Autodesk Inventor part; units mm, degrees
ref_plane "YZ Plane" through (0, 0, 0) normal (1, 0, 0) x (0, 1, 0)
ref_plane "XZ Plane" through (0, 0, 0) normal (0, 1, 0) x (-1, 0, 0)
ref_plane "XY Plane" through (0, 0, 0) normal (0, 0, 1) x (1, 0, 0)
sketch "スケッチ1" plane through (0, 0, 0) normal (0, 0, 1) x (1, 0, 0)
  circle A0 centre (295.848871, -93.120076) radius 1.5
  circle A1 centre (295.848871, -93.120076) radius 3.025
  line L0 (302.911618, -92.777137) -> (291.344796, -101.566309)
  arc A2 (282.40584, -101.176779) -> (291.344796, -101.566309) centre (287.109706, -95.992799) ccw
  arc A3 (299.078829, -95.689522) -> (299.346701, -89.542385) centre (296.658778, -92.504659) ccw
  line L1 (214.413679, -12.475426) -> (302.911618, -92.777137)
  line L2 (186.870748, -14.489658) -> (289.472001, -107.588508)
  line L3 (89.513673, -53) -> (377.048162, -53)
  circle A4 centre (295.848871, -93.120076) radius 4.025
  circle A5 centre (295.848871, -93.120076) radius 6
  line L4 (290.052231, -91.571215) -> (285.593636, -108.257588)
  circle A6 centre (285.42622, -97.165857) radius 3.025
  arc A7 (287.438666, -101.35253) -> (289.20342, -107.344802) centre (293.235305, -102.901391) ccw
  circle A8 centre (298.015884, -108.589531) radius 3
  circle A9 centre (298.015884, -108.589531) radius 1.5
  line L5 (185.106531, 0.614305) -> (481.333939, -268.178035)
  line L6 (295.848871, -93.120076) -> (289.20342, -100.443813) construction
  line L7 (301.069617, -90.163082) -> (333.637532, -147.663653)
  line L8 (333.637532, -147.663653) -> (289.20342, -107.344802)
  circle A10 centre (295.848871, -93.120076) radius 1.5
  circle A11 centre (295.848871, -93.120076) radius 3.025
  line L9 (302.911618, -92.777137) -> (291.344796, -101.566309)
  arc A12 (282.40584, -101.176779) -> (291.344796, -101.566309) centre (287.109706, -95.992799) ccw
  arc A13 (299.078829, -95.689522) -> (299.346701, -89.542385) centre (296.658778, -92.504659) ccw
  line L10 (214.413679, -12.475426) -> (302.911618, -92.777137)
  line L11 (186.870748, -14.489658) -> (289.472001, -107.588508)
  line L12 (89.513673, -53) -> (377.048162, -53)
  circle A14 centre (295.848871, -93.120076) radius 4.025
  circle A15 centre (295.848871, -93.120076) radius 6
  line L13 (290.052231, -91.571215) -> (285.593636, -108.257588)
  circle A16 centre (285.42622, -97.165857) radius 3.025
  arc A17 (287.438666, -101.35253) -> (289.20342, -107.344802) centre (293.235305, -102.901391) ccw
  circle A18 centre (298.015884, -108.589531) radius 3 construction
  circle A19 centre (298.015884, -108.589531) radius 1.5
  line L14 (185.106531, 0.614305) -> (481.333939, -268.178035)
  line L15 (295.848871, -93.120076) -> (289.20342, -100.443813) construction
  line L16 (301.069617, -90.163082) -> (333.637532, -147.663653)
  line L17 (333.637532, -147.663653) -> (289.20342, -107.344802)
  line L18 (301.984952, -108.140062) -> (343.184474, -145.523895)
  circle A20 centre (305.221577, -116.478183) radius 1.5
  circle A21 centre (316.330105, -126.557896) radius 1.5
  line L19 (301.984952, -108.140062) -> (293.498432, -117.492783)
  arc A22 (303.540146, -109.551222) -> (301.984952, -108.140062) centre (302.762549, -108.845642) ccw
  line L20 (301.984952, -108.140062) -> (302.762549, -108.845642) construction
  line L21 (303.540146, -109.551222) -> (302.762549, -108.845642) construction
  point P0 (0, 0)
  point P1 (0, 0)
  point P2 (297.912288, -96.575931)
  point P3 (298.625557, -96.033946)
  point P4 (0, 0)
  point P5 (296.609105, -114.064611)
  point P6 (321.049741, -125.439168)
  dimension "d0" = 8.05
  dimension "d1" = 12
  dimension "d2" = 6
  dimension "d3" = 6
  dimension "d4" = 3
  dimension "d5" = 5
  dimension "d6" = 12
  dimension "d7" = 60
  dimension "d11" = 8.05
  dimension "d12" = 12
  dimension "d13" = 6
  dimension "d14" = 6
  dimension "d15" = 3
  dimension "d16" = 5
  dimension "d17" = 12
  dimension "d18" = 60
  dimension "d19" = 8
  dimension "d20" = 4
  dimension "d21" = 4
  dimension "d22" = 3
  dimension "d23" = 50
  dimension "d24" = 8
  dimension "d25" = 15
  dimension "d28" = 1.05
  dimension "d29" = 180
extrude "押し出し1" add sketch "スケッチ1" along normal blind 5 contours L7 L5 A5 L0 | L0 A5 L1 L7 | L1 A5 L7 | A5 L5 L0 A4 | L0 A3 L1 A5 | L7 L18 A22 L19 A8 L8 L2 A7 A2 L0 A5 L5 | L1 A5 | L0 A4 L5 A5 L1 A3 | A5 L0 L5 | L7 L8 L19 A8 L18 | A4 L0 | A5 L5 L0 | L0 A2 A7 L4 L5 A5 | L18 A22 | A5 L5 L4 | L19 A8 | A8 L19 | A9 picked at (298.233704, -96.341002)
fillet "フィレット1" radius 1 1 edges at (333.6375, -147.6637, 2.5)
extrude "押し出し2" cut sketch "スケッチ1" along normal blind 2 contours L7 L8 L19 A8 L18 | L18 A22 | L19 A8 picked at (299.870596, -110.60445)
sketch "スケッチ2" plane through (0, 0, 5) normal (0, 0, 1) x (1, 0, 0)
  arc A0 (329.027651, -143.480716) -> (330.569756, -142.247316) centre (329.699632, -142.740148) ccw
  line L0 (330.569756, -142.247316) -> (301.069617, -90.163082)
  arc A1 (301.069617, -90.163082) -> (290.052231, -91.571215) centre (295.848871, -93.120076) ccw
  line L1 (290.052231, -91.571215) -> (287.438666, -101.35253)
  arc A2 (287.438666, -101.35253) -> (289.20342, -107.344802) centre (293.235305, -102.901391) ccw
  line L2 (289.20342, -107.344802) -> (329.027651, -143.480716)
  arc A3 (298.625557, -96.033946) -> (297.912288, -96.575931) centre (295.848871, -93.120076) ccw
  line L3 (298.625557, -96.033946) -> (297.912288, -96.575931)
  circle A4 centre (316.330105, -126.557896) radius 1.5
  circle A5 centre (305.221577, -116.478183) radius 1.5
  line L4 (301.984952, -108.140062) -> (296.609105, -114.064611)
  line L5 (289.20342, -107.344802) -> (296.609105, -114.064611)
  line L6 (293.646831, -111.376687) -> (291.510724, -104.715452)
  line L7 (295.412844, -104.007733) -> (295.868537, -113.39263)
  arc A6 (295.412844, -104.007733) -> (291.510724, -104.715452) centre (293.415198, -104.104731) ccw
  point P0 (0, 0)
  point P1 (293.646831, -111.376687)
  dimension "d31" = 30
  dimension "d32" = 45
  dimension "d33" = 3
  dimension "d34" = 2
  dimension "d37" = 1
extrude "押し出し3" cut sketch "スケッチ2" against normal blind 10 contours L2 L6 A6 L7
equation "\"d20\" = 0.5 * d19"
equation "\"d21\" = d20"
properties part number "アーム先端" material "ポリカーボネート、スモーク"
For this review, take the finished solid that the model builds, in its own axes (mm). A direction names the side the tool comes from. Give positions to 0.01 mm unless a question says otherwise; leave off trailing zeros. Order: outer loops, then holes, each group sorted by start corner. A loop starts at its lowest first (then second) coordinate and runs counter-clockwise, first axis right, second up. Notation, with made-up numbers: (-22.75, 4.5) - (24.25, 4.5) arc R3 ccw to (24.25, 8.5) - close; hole circle Ø5 at (59, 42.25). An arc over 180 degrees is marked (long way). Answer as a JSON object with one key per item and string values. Group by question number.
Item 1: Take a section at D-D on x = 311.5. Give the boundary of the cut face in (y, z), and give its area (3 significant figures).
Item 2: Clearance check with flat-ended pins moving along their axes: pin 1 Ø1.5 at (y, z) = (-112.5, 4) entering from -X; pin 2 Ø3 at (y, z) = (-130, 2) entering from -X; pin 3 Ø3.5 at (x, y) = (305.22, -116.48) entering from +Z; pin 4 Ø2 at (x, z) = (321.5, 0.5) entering from +Y. State where each tip first meets the part, or that it passes through.
Item 3: Draft analysis for pull direction X (two halves, no side actions). For faces 1 (the cylindrical face through (293.11, -102.13, 2.54)), 2 (the cylindrical face through (287.493, -104.641, 2.465)), 3 (the flat face through (312.335, -110.053, 2.465)), state which applies: pulls with the +X half, pulls with the -X half, needs draft (parallel to the pull), parting line crosses it, or undercut.
Item 4: Take a section at C-C on x = 305.5. Give the boundary of the cut face in (y, z).
Item 5: Machinability: for faces 4 (the cylindrical face through (303.5, -108.1, 1)), 5 (the flat face through (299.3, -111.1, 1)), 6 (the flat face through (295.638, -108.634, 2.535)), 7 (the flat face through (292.594, -108.093, 2.535)), which of the approach directions +Z, -Z, +X, -X, +Y, -Y give a long, thin tool a straight path to every point of the face, cutting with its end or side? Answer none if there is none.
Item 6: Take a section at B-B on y = -106.5. Give the boundary of the cut face in (x, z), and give its area (3 significant figures).
Item 7: Wall thickness on line 1 along Z through (x, y) = (311, -120.5); line 2 along Y through (x, z) = (294, 1.2); line 3 along Y through (x, z) = (305, 2.25): over which ranges is each line inside the solid? List them lowest first.
Reported:
{
 "1": {"outline": "(-127.58, 2) - (-116.77, 2) - (-116.77, 0) - (-108.58, 0) - (-108.58, 5) - (-127.58, 5) - close", "area": "73.4 mm^2"},
 "2": {"pin 1": "x = 295.79", "pin 2": "x = 312.52", "pin 3": "z = 5", "pin 4": "y = -124.47"},
 "3": {"face 1": "undercut", "face 2": "pulls with the -X half", "face 3": "pulls with the +X half"},
 "4": {"outline": "(-122.13, 2) - (-117.95, 2) - (-117.95, 5) - (-122.13, 5) - close; (-115, 2) - (-111.33, 2) - (-111.33, 0) - (-97.99, 0) - (-97.99, 5) - (-115, 5) - close"},
 "5": {"face 4": "-Z", "face 5": "-Z, -Y", "face 6": "+Z, -Z, -Y", "face 7": "+Z, -Z"},
 "6": {"outline": "(288.43, 0) - (292.08, 0) - (292.08, 5) - (288.43, 5) - close; (295.53, 0) - (310.32, 0) - (310.32, 5) - (295.53, 5) - close", "area": "92.2 mm^2"},
 "7": {"line 1": "2 to 5", "line 2": "-102.19 to -96.7, -89.54 to -87.41", "line 3": "-121.68 to -117.96, -114.99 to -97.1"}
}
